Can you work these out from the model? Positions are in its coordinate system, mm. Face numbers are marked on the shaded views. A direction names the side the tool comes from. Coordinates: 2 decimals unless noted, no trailing zeros. Order: outer loops, then holes, each group sorted by start corner. A loop starts at its lowest first (then second) coordinate and runs counter-clockwise, first axis right, second up. Notation, with made-up numbers: M 12,57.5 L 51,57.5 A10 cw 51,70.5 Z; hole C 31.5,19.25 d10. An arc over 180 degrees is marked long. Answer as CSV lines item,"result". Start each with the question number.
1. If we section it at B-B (x = 0): List the corners of the cut face in (y, z) for me, plus the area to 3 significant figures.
2. I need wall thicknesses on line 1 along Y through (x, z) = (-19, 29); line 2 along X through (y, z) = (4.75, 6); line 3 along Y through (x, z) = (0, 1.3). Which ranges of each line are inside material? Lowest first, please. Write a range as from..to.
3. If we section it at C-C (z = 28): List the corners of the cut face in (x, y) for me.
4. On a 3-axis mill with a long thin cutter (end or side, diameter ignored), from which of +Z, -Z, +X, -X, +Y, -Y can I reach the whole of each face in a straight line? I mean the marked faces 1, 2, 3, 4 and 5. Say none if no direction works.
5. Will these pins go through, and if not, where does the flat tip stop? pin 1 (5 mm diameter, centred on y = 0, z = 14.5, fed in from +X); pin 2 (6 mm diameter, centred on x = -5.5, y = -2.5, fed in from -Z); pin 3 (4.5 mm diameter, centred on x = -18, y = 3, fed in from -Z); pin 4 (8 mm diameter, centred on y = -4.5, z = 16.5, fed in from -X).
6. If we section it at D-D (x = -16): List the corners of the cut face in (y, z) for me, plus the area to 4 significant figures.
7. If we mould it in two halves opening along Y, with no side actions, what happens to the marked faces 6, 7, 8 and 9? For each: released by +Y, released by -Y, zero draft, split by the parting line, or undercut.
8. If we section it at A-A (y = 5): List the corners of the cut face in (x, z) for me.
```python
from build123d import *

# Parameters (mm, degrees)
SKETCH1_W           = 20
SKETCH1_H           = 16
SKETCH1_R           = 6.25
BOSS_EXTRUDE1_DEPTH = 5
SKETCH2_W           = 3
SKETCH2_H           = 16
BOSS_EXTRUDE2_DEPTH = 26
SKETCH3_W           = 18
SKETCH3_H           = 16
BOSS_EXTRUDE3_DEPTH = 2.5
CUT_EXTRUDE1_DEPTH  = 39.745967532


with BuildPart() as part:
    # Sketch1 → Boss-Extrude1 (new body)
    with BuildSketch(Plane.XY):
        Rectangle(SKETCH1_W, SKETCH1_H)
        Circle(SKETCH1_R, mode=Mode.SUBTRACT)
    extrude(amount=BOSS_EXTRUDE1_DEPTH)

    # Sketch2 → Boss-Extrude2 (add)
    with BuildSketch(Plane.XY.offset(5)):
        with Locations((-8.5, 0)):
            Rectangle(SKETCH2_W, SKETCH2_H)
        with Locations((8.5, 0)):
            Rectangle(SKETCH2_W, SKETCH2_H)
    extrude(amount=BOSS_EXTRUDE2_DEPTH)

    # Sketch3 → Boss-Extrude3 (add)
    with BuildSketch(Plane.XY.offset(31)):
        with Locations((-16, 0)):
            Rectangle(SKETCH3_W, SKETCH3_H)
        with Locations((16, 0)):
            Rectangle(SKETCH3_W, SKETCH3_H)
    extrude(amount=-BOSS_EXTRUDE3_DEPTH)

    # Sketch4 → Cut-Extrude1 (cut, through all)
    with BuildSketch(Plane(origin=(0, 0, 28.5), x_dir=(-1, 0, 0), z_dir=(0, 0, -1))):
        with BuildLine():
            Line((-22.5, -3.25), (-12.5, -3.25))
            ThreePointArc((-12.5, -3.25), (-10.75, -5), (-12.5, -6.75))
            Line((-12.5, -6.75), (-22.5, -6.75))
            ThreePointArc((-22.5, -6.75), (-24.25, -5), (-22.5, -3.25))
        make_face()
        with BuildLine():
            Line((22.5, 6.75), (12.5, 6.75))
            ThreePointArc((12.5, 6.75), (10.75, 5), (12.5, 3.25))
            Line((12.5, 3.25), (22.5, 3.25))
            ThreePointArc((22.5, 3.25), (24.25, 5), (22.5, 6.75))
        make_face()
        with BuildLine():
            Line((-22.5, 1.75), (-12.5, 1.75))
            ThreePointArc((-12.5, 1.75), (-10.75, 0), (-12.5, -1.75))
            Line((-12.5, -1.75), (-22.5, -1.75))
            ThreePointArc((-22.5, -1.75), (-24.25, 0), (-22.5, 1.75))
        make_face()
        with BuildLine():
            Line((-22.5, 6.75), (-12.5, 6.75))
            ThreePointArc((-12.5, 6.75), (-10.75, 5), (-12.5, 3.25))
            Line((-12.5, 3.25), (-22.5, 3.25))
            ThreePointArc((-22.5, 3.25), (-24.25, 5), (-22.5, 6.75))
        make_face()
        with BuildLine():
            Line((22.5, 1.75), (12.5, 1.75))
            ThreePointArc((12.5, 1.75), (10.75, 0), (12.5, -1.75))
            Line((12.5, -1.75), (22.5, -1.75))
            ThreePointArc((22.5, -1.75), (24.25, 0), (22.5, 1.75))
        make_face()
        with BuildLine():
            Line((22.5, -3.25), (12.5, -3.25))
            ThreePointArc((12.5, -3.25), (10.75, -5), (12.5, -6.75))
            Line((12.5, -6.75), (22.5, -6.75))
            ThreePointArc((22.5, -6.75), (24.25, -5), (22.5, -3.25))
        make_face()
    extrude(amount=-CUT_EXTRUDE1_DEPTH, mode=Mode.SUBTRACT)


solid = part.part
```
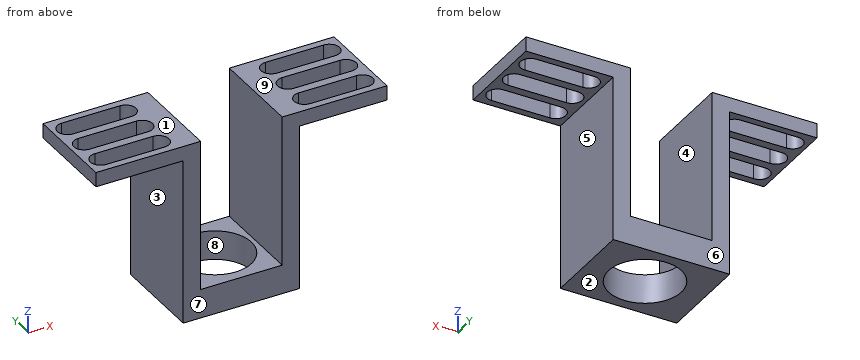
Solved:
1,outline,"M -8,0 L -6.25,0 L -6.25,5 L -8,5 Z; M 6.25,0 L 8,0 L 8,5 L 6.25,5 Z"
1,area,"17.5 mm²"
2,line 1,"-8..-6.75, -3.25..-1.75, 1.75..3.25, 6.75..8"
2,line 2,"-10..-7, 7..10"
2,line 3,"-8..-6.25, 6.25..8"
3,outline,"M -10,-8 L -7,-8 L -7,8 L -10,8 Z; M 7,-8 L 10,-8 L 10,8 L 7,8 Z"
4,face 1,"+Z, +X, -X, +Y, -Y"
4,face 2,"-Z, +X, -X, +Y, -Y"
4,face 3,"-Z, -X, +Y, -Y"
4,face 4,"+Z, +Y, -Y"
4,face 5,"-Z, +X, +Y, -Y"
5,pin 1,"x = 10"
5,pin 2,"z = 0"
5,pin 3,"z = 28.5"
5,pin 4,"x = -10"
6,outline,"M -8,28.5 L -6.75,28.5 L -6.75,31 L -8,31 Z; M -3.25,28.5 L -1.75,28.5 L -1.75,31 L -3.25,31 Z; M 1.75,28.5 L 3.25,28.5 L 3.25,31 L 1.75,31 Z; M 6.75,28.5 L 8,28.5 L 8,31 L 6.75,31 Z"
6,area,"13.75 mm²"
7,face 6,"released by +Y"
7,face 7,"released by -Y"
7,face 8,"undercut"
7,face 9,"zero draft"
8,outline,"M -25,28.5 L -24.25,28.5 L -24.25,31 L -25,31 Z; M -10.75,28.5 L -10,28.5 L -10,0 L -3.75,0 L -3.75,5 L -7,5 L -7,31 L -10.75,31 Z; M 3.75,0 L 10,0 L 10,28.5 L 10.75,28.5 L 10.75,31 L 7,31 L 7,5 L 3.75,5 Z; M 24.25,28.5 L 25,28.5 L 25,31 L 24.25,31 Z"
